```python
from build123d import *

# Parameters (mm, degrees)
SKETCH_R        = 9.5
SKETCH_R_2      = 1.75
PAD_DEPTH       = 5
POCKET_DEPTH    = 3
SKETCH002_R     = 1.625
POCKET001_DEPTH = 5.001
SKETCH003_R     = 2.875
POCKET002_DEPTH = 4.5
CHAMFER_SIZE    = 1
CHAMFER002_SIZE = 0.5


with BuildPart() as part:
    # Sketch → Pad (new body)
    with BuildSketch(Plane.XY):
        with BuildLine():
            Line((16.75, 21), (21, 17.433827))
            Line((21, 17.433827), (21, 0))
            Line((21, -17.433827), (21, 0))
            Line((16.75, -21), (21, -17.433827))
            Line((16.75, -21), (9.5, -21))
            ThreePointArc((9.5, -21), (0, -11.5), (-9.5, -21))
            Line((-16.75, -21), (-9.5, -21))
            Line((-21, -17.433827), (-16.75, -21))
            Line((-21, 0), (-21, -17.433827))
            Line((-21, 17.433827), (-21, 0))
            Line((-16.75, 21), (-21, 17.433827))
            Line((-16.75, 21), (-9.5, 21))
            ThreePointArc((-9.5, 21), (0, 11.5), (9.5, 21))
            Line((9.5, 21), (16.75, 21))
        make_face()
        Circle(SKETCH_R, mode=Mode.SUBTRACT)
        with Locations((-15.5, 15.5)):
            Circle(SKETCH_R_2, mode=Mode.SUBTRACT)
        with Locations((15.5, 15.5)):
            Circle(SKETCH_R_2, mode=Mode.SUBTRACT)
        with Locations((-15.5, -15.5)):
            Circle(SKETCH_R_2, mode=Mode.SUBTRACT)
        with Locations((15.5, -15.5)):
            Circle(SKETCH_R_2, mode=Mode.SUBTRACT)
    extrude(amount=PAD_DEPTH)

    # Sketch001 → Pocket (cut)
    with BuildSketch(Plane.XY):
        Polygon((-15.5, 4.2), (-12.642116, 5.85), (-12.642116, 9.15), (-15.5, 10.8), (-18.357884, 9.15), (-18.357884, 5.85), align=None)
        Polygon((-12.642116, -9.15), (-12.642116, -5.85), (-15.5, -4.2), (-18.357884, -5.85), (-18.357884, -9.15), (-15.5, -10.8), align=None)
        Polygon((18.357884, 5.85), (18.357884, 9.15), (15.5, 10.8), (12.642116, 9.15), (12.642116, 5.85), (15.5, 4.2), align=None)
        Polygon((18.357884, -9.15), (18.357884, -5.85), (15.5, -4.2), (12.642116, -5.85), (12.642116, -9.15), (15.5, -10.8), align=None)
    extrude(amount=POCKET_DEPTH, mode=Mode.SUBTRACT)

    # Sketch002 → Pocket001 (cut, through all)
    with BuildSketch(Plane.XY):
        with Locations((-15.5, 7.5)):
            Circle(SKETCH002_R)
        with Locations((15.5, 7.5)):
            Circle(SKETCH002_R)
        with Locations((15.5, -7.5)):
            Circle(SKETCH002_R)
        with Locations((-15.5, -7.5)):
            Circle(SKETCH002_R)
    extrude(amount=POCKET001_DEPTH, mode=Mode.SUBTRACT)

    # Sketch003 → Pocket002 (cut)
    with BuildSketch(Plane.XY.offset(5)):
        with Locations((-15.5, 15.5)):
            Circle(SKETCH003_R)
        with Locations((15.5, 15.5)):
            Circle(SKETCH003_R)
        with Locations((-15.5, -15.5)):
            Circle(SKETCH003_R)
        with Locations((15.5, -15.5)):
            Circle(SKETCH003_R)
    extrude(amount=-POCKET002_DEPTH, mode=Mode.SUBTRACT)

    # Chamfer
    chamfer_edges = [part.edges().sort_by_distance(p)[0] for p in [
        (-13.125, -21, 5),
        (-18.875, -19.216913, 5),
        (-21, -8.716913, 5),
        (-21, 8.716913, 5),
        (-18.875, 19.216913, 5),
        (-13.125, 21, 5),
        (0, 11.5, 5),
        (13.125, 21, 5),
        (18.875, 19.216913, 5),
        (21, 8.716913, 5),
        (21, -8.716913, 5),
        (0, -11.5, 5),
        (13.125, -21, 5),
        (18.875, -19.216913, 5),
    ]]
    chamfer(chamfer_edges, length=CHAMFER_SIZE)

    # Chamfer002
    chamfer002_edges = [part.edges().sort_by_distance(p)[0] for p in [
        (-9.5, 0, 5),
    ]]
    chamfer(chamfer002_edges, length=CHAMFER002_SIZE)


solid = part.part
```
Check sheet for the modelled part. Datum: model origin and axes. Units: mm. A direction names the side the tool comes from. Round coordinates to 2 decimals unless told otherwise and drop trailing zeros.
1) Mould release check, pull along Y, two halves, no side actions. Record for faces 1 (the cylindrical face through (-0.209, 11.502, 1.972)), 2 (the flat face through (18.358, 7, 1)), 3 (the flat face through (-18.905, -19.192, 1.972)): +Y half, -Y half, draft (parallel to the pull), parting line (faces both ways), or undercut.
2) Scan lines: line 1 (Y direction, x = 15.5, z = 0.25); line 2 (Y direction, x = -15.5, z = 1.7) (3 decimals); line 3 (X direction, y = 15.5, z = 0.4). Record each from-to range of solid material in increasing order.
3) Section check A-A (y = -7.5). Give the number of separate pieces and of enclosed holes in the cut face, and give its area (3 significant figures).
4) Tool access check on faces 4 (the flat face through (-14.051, -5.037, 1.479)), 5 (the flat face through (-18.85, 19.24, 1.97)), 6 (the flat face through (17, -17, 0.5)). Record the directions out of +Z, -Z, +X, -X, +Y, -Y that give a thin tool (end or side, any length) a straight path to the whole face; none if there is none.
5) Go/stop test with flat-tipped pins: pin 1 Ø4.5 at (x, y) = (-15.5, -15.5) entering from +Z; pin 2 Ø1.7 at (x, y) = (17, -7) entering from -Z. Record where each tip stops, or that it passes through.
Result:
1. face 1: +Y half
1. face 2: undercut
1. face 3: -Y half
2. line 1: y = -21 to -17.25, -13.75 to -10.8, -4.2 to 4.2, 10.8 to 13.75, 17.25 to 21
2. line 2: y = -21 to -18.375, -12.625 to -10.8, -4.2 to 4.2, 10.8 to 12.625, 18.375 to 21
2. line 3: x = -21 to -17.25, -13.75 to -7.75, 7.75 to 13.75, 17.25 to 21
3. separate pieces: 4
3. enclosed holes: 0
3. area: 103 mm2
4. face 4: -Z
4. face 5: +Z, -Z, -X, +Y
4. face 6: +Z
5. pin 1: stops at z = 0.5
5. pin 2: stops at z = 3
